Part model, mm, in its own coordinate system. Face numbers are marked on the shaded views. A direction names the side the tool comes from. Round coordinates to 2 decimals unless told otherwise and drop trailing zeros. Loops run counter-clockwise (first coordinate to the right, second up) from the corner with the lowest first, then second, coordinate; pieces in that order, holes last. Notation, with made-up numbers: (-27.75, 20.5) - (-10.75, 20.5) arc R24 ccw to (-10.75, 33.5) - close; hole circle Ø11 at (-31, 7.5). An arc over 180 degrees is marked (long way). Write each question's results on one line, items separated by ' | '. Start each with the question number.
(1) Cut at D-D, the plane x = 20. List the corners of the cut face in (y, z), then the cut area to 3 significant figures.
(2) Drill centre lines: L1, parallel to X at y = -2.1, z = 10; L2, parallel to Z at x = 0.75, y = -20; L3, parallel to X at y = -28, z = 5.25. Where is each one in solid material? Low to high.
(3) Flat gauge pins, fed straight in: P1, Ø1.2, axis at x = -0.5, y = -7.5, coming from the +Z side; P2, Ø0.9, axis at y = 0.5, z = 10.5, coming from the -X side; P3, Ø10, axis at x = 14.5, y = -19, coming from the +Z side; P4, Ø4, axis at y = -19.5, z = 17, coming from the +X side. Where does each tip first touch, or does it go through?
(4) Cut at C-C, the plane z = 2.5. List the corners of the cut face in (x, y), then the cut area to 4 significant figures.
(5) Tool access for the marked faces 1 and 2: list every direction of +Z, -Z, +X, -X, +Y, -Y with a clear straight run to the whole face (end or side of a thin tool).
(6) Cut at A-A, the plane y = -2.5. List the corners of the cut face in (x, z), then the cut area to 3 significant figures.
(7) Mould opens along Z. For the marked faces 3, 4 and 5 say: released by +Z, released by -Z, zero draft, split by the parting line, or undercut.
(8) Cut at B-B, the plane y = -33. List the corners of the cut face in (x, z).
from build123d import *

# Parameters (mm, degrees)
BOSS_EXTRUDE1_DEPTH = 3.5
BOSS_EXTRUDE2_DEPTH = 16.5
BOSS_EXTRUDE3_DEPTH = 2.5
SKETCH4_R           = 2.2
CUT_EXTRUDE1_DEPTH  = 53.773099208
SKETCH5_R           = 2.2
CUT_EXTRUDE2_DEPTH  = 53.773099208
BOSS_EXTRUDE5_DEPTH = 36
SKETCH7_W           = 15
SKETCH7_H           = 1.1
CUT_EXTRUDE3_DEPTH  = 53.496095093
BOSS_EXTRUDE6_REACH = 57.429
SKETCH9_W           = 1.1
SKETCH9_H           = 15
CUT_EXTRUDE4_DEPTH  = 53.496095093
BOSS_EXTRUDE7_START = -12.383093
BOSS_EXTRUDE7_DEPTH = 12.383093
CUT_EXTRUDE5_DEPTH  = 60.161910074
CUT_EXTRUDE6_DEPTH  = 55.699177325


with BuildPart() as part:
    # Sketch1 → Boss-Extrude1 (new body)
    with BuildSketch(Plane.XY):
        Polygon((0, -36), (0, 0), (36, 0), (36, -3), (3, -36), align=None)
    extrude(amount=BOSS_EXTRUDE1_DEPTH)

    # Sketch2 → Boss-Extrude2 (add)
    with BuildSketch(Plane.XY.offset(3.5)):
        Polygon((0, -36), (0, 0), (36, 0), (36, -3), (3, -3), (3, -36), align=None)
    extrude(amount=BOSS_EXTRUDE2_DEPTH)

    # Sketch3 → Boss-Extrude3 (add)
    with BuildSketch(Plane.XY.offset(20)):
        Polygon((3, -21.5), (21.5, -3), (3, -3), align=None)
    extrude(amount=-BOSS_EXTRUDE3_DEPTH)

    # Sketch4 → Cut-Extrude1 (cut, through all)
    with BuildSketch(Plane.XZ.offset(3)):
        with Locations(Location((20, 10, 0), (0, 0, 270))):
            Circle(SKETCH4_R)
    extrude(amount=-CUT_EXTRUDE1_DEPTH, mode=Mode.SUBTRACT)

    # Sketch5 → Cut-Extrude2 (cut, through all)
    with BuildSketch(Plane(origin=(3, 0, 0), x_dir=(0, 0, -1), z_dir=(1, 0, 0))):
        with Locations((-10, -20)):
            Circle(SKETCH5_R)
    extrude(amount=-CUT_EXTRUDE2_DEPTH, mode=Mode.SUBTRACT)

    # Sketch6 → Boss-Extrude5 (add, through all)
    with BuildSketch(Plane(origin=(36, 0, 0), x_dir=(0, 0, -1), z_dir=(1, 0, 0))):
        Polygon((-12.8, 0), (-12.8, 1.1), (-9.6, 1.1), (-8.2, 0), align=None)
    extrude(amount=-BOSS_EXTRUDE5_DEPTH)

    # Sketch7 → Cut-Extrude3 (cut, through all)
    with BuildSketch(Plane.XY.offset(12.8)):
        with Locations((17.5, 0.55)):
            Rectangle(SKETCH7_W, SKETCH7_H)
    extrude(amount=-CUT_EXTRUDE3_DEPTH, mode=Mode.SUBTRACT)

    # Boss-Extrude6: up to this face of the body (flat: up to its plane)
    boss_extrude6_end = Plane(part.part.faces().sort_by_distance((0.411825206, 0, 16.4))[0])
    # Sketch8 → Boss-Extrude6 (add, up to the picked face)
    with BuildSketch(Plane.XZ.offset(36), mode=Mode.PRIVATE) as boss_extrude6_sk1:
        Polygon((0, 8.2), (0, 12.8), (-1.1, 12.8), (-1.1, 9.6), align=None)
    boss_extrude6_tool1 = split(extrude(boss_extrude6_sk1.sketch, amount=-BOSS_EXTRUDE6_REACH, mode=Mode.PRIVATE), bisect_by=boss_extrude6_end, keep=Keep.BOTH, mode=Mode.PRIVATE)
    add(boss_extrude6_tool1.solids().sort_by(Axis((-0.517094, -36, 10.82906), (0, 1, 0)))[0])

    # Sketch9 → Cut-Extrude4 (cut, through all)
    with BuildSketch(Plane.XY.offset(12.8)):
        with Locations((-0.55, -17.5)):
            Rectangle(SKETCH9_W, SKETCH9_H)
    extrude(amount=-CUT_EXTRUDE4_DEPTH, mode=Mode.SUBTRACT)

    # Sketch11 → Boss-Extrude7 (add)
    with BuildSketch(Plane(origin=(-2.016949153, 2.016949153, 4.389830508), x_dir=(-0.9228036153935797, -0.16085056987258428, -0.35008653442856574), z_dir=(0.3852706677344363, -0.38527066773443636, -0.8385302768337725)).offset(BOSS_EXTRUDE7_START)):
        Polygon((-25.484240374, -10.032283534), (-5.436637946, -26.842805147), (-5.436637946, -6.483532076), align=None)
    extrude(amount=BOSS_EXTRUDE7_DEPTH)

    # Sketch12 → Cut-Extrude5 (cut, through all)
    with BuildSketch(Plane(origin=(36, 0, 0), x_dir=(0, 0, -1), z_dir=(1, 0, 0))):
        Polygon((-20, 0), (-20, -21.5), (-27.88359819, -21.5), (-27.88359819, 1.770842411), (-14.747015728, 1.770842411), (-14.747015728, 0), align=None)
    extrude(amount=-CUT_EXTRUDE5_DEPTH, mode=Mode.SUBTRACT)

    # Sketch13 → Cut-Extrude6 (cut, through all)
    with BuildSketch(Plane(origin=(0, 0, 0), x_dir=(1, 0, 0), z_dir=(0, 1, 0))):
        Polygon((0, -15.529411765), (0, -20), (-1.6960193, -20), align=None)
    extrude(amount=-CUT_EXTRUDE6_DEPTH, mode=Mode.SUBTRACT)


solid = part.part
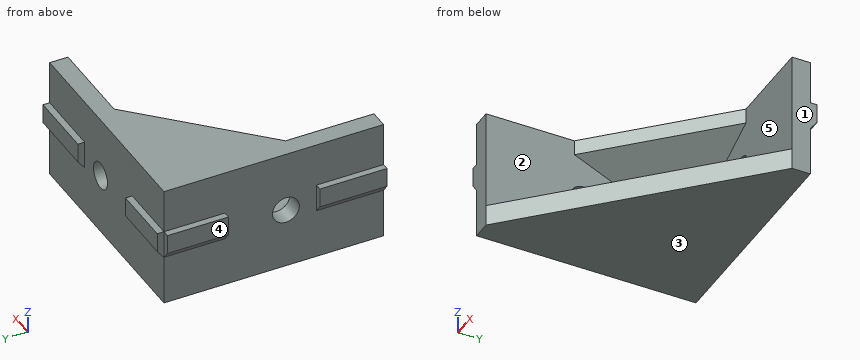
A:
1) outline: (-19, 0) - (0, 0) - (0, 7.8) - (-3, 7.8) - (-3, 3.5) - (-19, 3.5) - close; (-4.5, 17.5) - (-3, 16.81) - (-3, 12.2) - (0, 12.2) - (0, 20) - (-4.5, 20) - close | area: 107 mm2
2) L1: -1.1 to 17.8, 22.2 to 36 | L2: 0 to 7.8, 12.2 to 20 | L3: 0 to 3
3) P1: z = 20 | P2: x = 0 | P3: z = 3.5 | P4: x = 6.94
4) outline: (0, -36) - (3, -36) - (36, -3) - (36, 0) - (0, 0) - close | area: 751.5 mm2
5) face 1: +Z, -Z, +X, +Y, -Y | face 2: +X, -Y
6) outline: (-1.1, 9.6) - (0, 8.2) - (0, 0) - (36, 0) - (36, 20) - (0, 20) - (0, 12.8) - (-1.1, 12.8) - close; hole circle Ø4.4 at (20, 10) | area: 709 mm2
7) face 3: released by -Z | face 4: zero draft | face 5: undercut
8) outline: (-1.1, 9.6) - (0, 8.2) - (0, 0) - (6, 0) - (6, 3.5) - (3, 3.5) - (3, 20) - (0, 20) - (0, 12.8) - (-1.1, 12.8) - close
